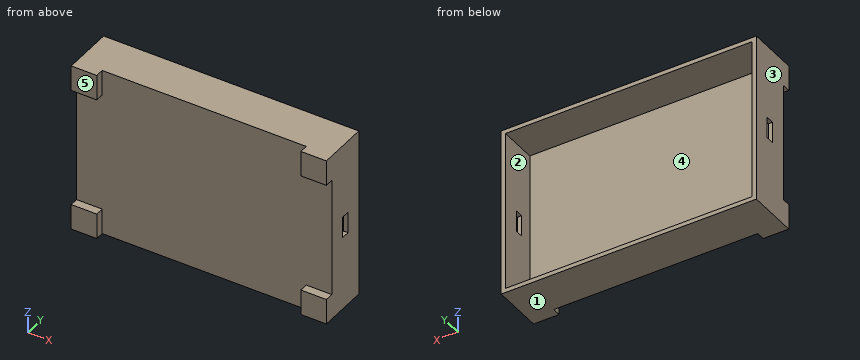
```python
from build123d import *

# Parameters (mm, degrees)
CROQUIS1_W              = 60
CROQUIS1_H              = 40
SALIENTE_EXTRUIR1_DEPTH = 10
VACIADO3_T              = -1
CROQUIS3_W              = 5
CROQUIS3_H              = 2
CORTAR_EXTRUIR1_DEPTH   = 65.031242374
CROQUIS4_W              = 6
CROQUIS4_H              = 6
SALIENTE_EXTRUIR2_DEPTH = 2


with BuildPart() as part:
    # Croquis1 → Saliente-Extruir1 (new body)
    with BuildSketch(Plane(origin=(0, 0, 0), x_dir=(1, 0, 0), z_dir=(0, 1, 0))):
        Rectangle(CROQUIS1_W, CROQUIS1_H)
    extrude(amount=SALIENTE_EXTRUIR1_DEPTH)

    # Vaciado3
    vaciado3_openings = [part.faces().sort_by_distance(p)[0] for p in [
        (0, 10, 0),
    ]]
    offset(amount=VACIADO3_T, openings=vaciado3_openings, kind=Kind.INTERSECTION)

    # Croquis3 → Cortar-Extruir1 (cut, through all)
    with BuildSketch(Plane.ZY.offset(30)):
        with Locations((0, 5)):
            Rectangle(CROQUIS3_W, CROQUIS3_H)
    extrude(amount=-CORTAR_EXTRUIR1_DEPTH, mode=Mode.SUBTRACT)

    # Croquis4 → Saliente-Extruir2 (add)
    with BuildSketch(Plane.XZ):
        with Locations((-27, 17)):
            Rectangle(CROQUIS4_W, CROQUIS4_H)
        with Locations((-27, -17)):
            Rectangle(CROQUIS4_W, CROQUIS4_H)
        with Locations((27, -17)):
            Rectangle(CROQUIS4_W, CROQUIS4_H)
        with Locations((27, 17)):
            Rectangle(CROQUIS4_W, CROQUIS4_H)
    extrude(amount=SALIENTE_EXTRUIR2_DEPTH)


solid = part.part
```
Here's how the part is built. I have some questions about the finished solid (model axes, mm). Face numbers are marked on the shaded views. A direction names the side the tool comes from. Coordinates: 2 decimals unless noted, no trailing zeros. Order: outer loops, then holes, each group sorted by start corner. A loop starts at its lowest first (then second) coordinate and runs counter-clockwise, first axis right, second up.
Item 1: If we section it at B-B, the plane y = 9: List the corners of the cut face in (x, z) for me, then the cut area to 3 significant figures.
Response values:
outline: (-30, -20) - (30, -20) - (30, 20) - (-30, 20) - close; hole (-29, -19) - (29, -19) - (29, 19) - (-29, 19) - close
area: 196 mm2
Item 2: I need wall thicknesses on probe 1 along X at (y, z) = (9, 2.5); probe 2 along Z at (x, y) = (-20.5, 2.5); probe 3 along Y at (x, z) = (9, -3). Which ranges of each line are inside material? Lowest first, please.
Response values:
probe 1: x = -30 to -29, 29 to 30
probe 2: z = -20 to -19, 19 to 20
probe 3: y = 0 to 1
Item 3: If we section it at C-C, the plane x = -13: List the corners of the cut face in (y, z) for me.
Response values:
outline: (0, -20) - (10, -20) - (10, -19) - (1, -19) - (1, 19) - (10, 19) - (10, 20) - (0, 20) - close
Item 4: Thinking about a two-plate mould opening in X: for the marked faces 3, 4 and 5, which applies, pulls with the +X half, pulls with the -X half, needs draft (parallel to the pull), parting line crosses it, or undercut?
Response values:
face 3: pulls with the -X half
face 4: undercut
face 5: needs draft
Item 5: Which directions (+Z, -Z, +X, -X, +Y, -Y) give clear straight access to the entire face, cutting with the end or side of a thin tool? Please do the marked faces 1 and 2.
Response values:
face 1: -Z, +X, -X, +Y, -Y
face 2: +Y
Item 6: If we section it at A-A, the plane z = -0.5: List the corners of the cut face in (x, y) for me.
Response values:
outline: (-30, 0) - (30, 0) - (30, 4) - (29, 4) - (29, 1) - (-29, 1) - (-29, 4) - (-30, 4) - close; (-30, 6) - (-29, 6) - (-29, 10) - (-30, 10) - close; (29, 6) - (30, 6) - (30, 10) - (29, 10) - close
Item 7: I'm going to push flat-ended pins straight in: pin 1 Ø5 at (x, z) = (8, -15) entering from +Y; pin 2 Ø1.5 at (x, z) = (-22.5, -5.5) entering from -Y. Where does each tip first touch, or does it pass through?
Response values:
pin 1: stops at y = 1
pin 2: stops at y = 0
Item 8: If we section it at D-D, the plane z = 17: List the corners of the cut face in (x, y) for me, then the cut area to 3 significant figures.
Response values:
outline: (-30, -2) - (-24, -2) - (-24, 0) - (24, 0) - (24, -2) - (30, -2) - (30, 10) - (29, 10) - (29, 1) - (-29, 1) - (-29, 10) - (-30, 10) - close
area: 102 mm2
